Part model, mm, in its own coordinate system. A direction names the side the tool comes from. Give positions to 0.01 mm unless a question says otherwise; leave off trailing zeros. Order: outer loops, then holes, each group sorted by start corner. A loop starts at its lowest first (then second) coordinate and runs counter-clockwise, first axis right, second up. Notation, with made-up numbers: (-24, -12.5) - (22, -12.5) arc R37 ccw to (22, 23.5) - close; hole circle Ø3 at (31, 37). An arc over 180 degrees is marked (long way). Use one line per item in the form item = value. Start each with the question number.
1. Band-saw the part on B-B, the plane y = -25.5. List the corners of the cut face in (x, z), plus the area to 3 significant figures.
2. Band-saw the part on D-D, the plane x = 30. List the corners of the cut face in (y, z), plus the area to 3 significant figures.
3. Drill centre lines: line 1 (X direction, y = -22.25, z = 0); line 2 (Z direction, x = -30, y = -22.5); line 3 (Z direction, x = 0, y = 4). Where is each one in solid material? Low to high.
4. Band-saw the part on A-A, the plane x = 0. List the corners of the cut face in (y, z).
5. Band-saw the part on C-C, the plane y = 88.5. List the corners of the cut face in (x, z), plus the area to 3 significant figures.
6. Pin check, flat tips, straight feed: P1, Ø8, axis at x = 9, z = 7.5, coming from the +Y side; P2, Ø2, axis at y = 36, z = 10.5, coming from the -X side; P3, Ø6, axis at x = -23.5, z = 4.5, coming from the +Y side; P4, Ø1, axis at y = 74.5, z = 13, coming from the +X side. Stop position of each tip, or through.
7. Tool access for faces 1 (the face through (-13.887, 2.086, 10.648)), 2 (the face through (31, -24, -10)), 3 (the face through (-31, -24, 10)), 4 (the face through (-30, -24, -10)): list every direction of +Z, -Z, +X, -X, +Y, -Y with a clear straight run to the whole face (end or side of a thin tool).
from build123d import *

# Parameters (mm, degrees)
SKETCH1_R           = 17.5
SKETCH1_R_2         = 12.75
BOSS_EXTRUDE1_DEPTH = 149
SKETCH3_R           = 3.25
BOSS_EXTRUDE2_DEPTH = 10


with BuildPart() as part:
    # Sketch1 → Boss-Extrude1 (new body, symmetric)
    with BuildSketch(Plane(origin=(0, 0, 0), x_dir=(1, 0, 0), z_dir=(0, 1, 0))):
        Circle(SKETCH1_R)
        Circle(SKETCH1_R_2, mode=Mode.SUBTRACT)
    extrude(amount=BOSS_EXTRUDE1_DEPTH, both=True)

    # Sketch3 → Boss-Extrude2 (add)
    with BuildSketch(Plane(origin=(0, -29, 0), x_dir=(-1, 0, 0), z_dir=(0, -1, 0))):
        with BuildLine():
            Line((47, -10), (7.90964601, -10))
            ThreePointArc((7.90964601, -10), (12.75, 0), (7.90964601, 10))
            Line((7.90964601, 10), (47, 10))
            Line((47, 10), (47, -10))
        make_face()
        with Locations((30, 0)):
            Circle(SKETCH3_R, mode=Mode.SUBTRACT)
        with BuildLine():
            Line((-47, -10), (-47, 10))
            Line((-47, 10), (-7.90964601, 10))
            ThreePointArc((-7.90964601, 10), (-12.75, 0), (-7.90964601, -10))
            Line((-7.90964601, -10), (-47, -10))
        make_face()
        with Locations((-30, 0)):
            Circle(SKETCH3_R, mode=Mode.SUBTRACT)
    extrude(amount=-BOSS_EXTRUDE2_DEPTH)


solid = part.part
From the geometry:
q1.outline = (-47, -10) - (-14.36, -10) arc R17.5 ccw to (14.36, -10) - (47, -10) - (47, 10) - (14.36, 10) arc R17.5 ccw to (-14.36, 10) - (-47, 10) - close; hole circle Ø6.5 at (-30, 0); hole circle Ø25.5 at (0, 0); hole circle Ø6.5 at (30, 0)
q1.area = 1,610 mm²
q2.outline = (-29, -10) - (-19, -10) - (-19, -3.25) - (-29, -3.25) - close; (-29, 3.25) - (-19, 3.25) - (-19, 10) - (-29, 10) - close
q2.area = 135 mm²
q3.line_1 = -47 to -33.25, -26.75 to -12.75, 12.75 to 26.75, 33.25 to 47
q3.line_2 = -10 to -3.25, 3.25 to 10
q3.line_3 = -17.5 to -12.75, 12.75 to 17.5
q4.outline = (-149, -17.5) - (149, -17.5) - (149, -12.75) - (-149, -12.75) - close; (-149, 12.75) - (149, 12.75) - (149, 17.5) - (-149, 17.5) - close
q5.outline = circle Ø35 at (0, 0); hole circle Ø25.5 at (0, 0)
q5.area = 451 mm²
q6.P1 = 149
q6.P2 = -14.7
q6.P3 = -19
q6.P4 = 12.25
q7.face_1 = none
q7.face_2 = -Z, +X, +Y, -Y
q7.face_3 = +Z, -X, +Y, -Y
q7.face_4 = -Z, -X, +Y, -Y
